Answer from the drawing. Dimensions are ordinates in mm from the lowest x, y and z of the part. A direction names the side the tool comes from. Coordinates: 2 decimals unless noted, no trailing zeros. Write each loop counter-clockwise with the first axis right and the second up, starting at its lowest first coordinate (ties: lowest second). Pieces come first, ordered by that corner, then holes.
(1) The part is cut by section B-B, the plane y = 42.5. Determine the outline of the cut face in (x, z) (1 decimal).
(2) Which of the six approach directions +Z, -Z, +X, -X, +Y, -Y give full straight-line access (tool end or side, diameter ignored) to the marked faces 5 and 6?
(3) The part is cut by section A-A, the plane z = 26.5. Determine the outline of the cut face in (x, y) (1 decimal).
(4) Straight lines are drawn through the part: line 1 along X through (y, z) = (20, 48) (1 decimal); line 2 along Y through (x, z) = (11, 48) (1 decimal); line 3 along Z through (x, y) = (25, 26). For each, find the intervals that lie inside material, in ascending order.
(5) Given pin 1 (5 mm diameter, centred on x = 21.5, y = 18, fed in from +Z), flat-ended and moving along its own axis, determine where the tip first touches the part or whether it passes through.
(6) The part is cut by section C-C, the plane x = 3. Determine the outline of the cut face in (y, z) (1 decimal), and give its area (3 significant figures).
(7) Determine the mould class of the marked faces 1, 2, 3 and 4 for opening direction Y: pulls with the +Y half, pulls with the -Y half, needs draft (parallel to the pull), parting line crosses it, or undercut.
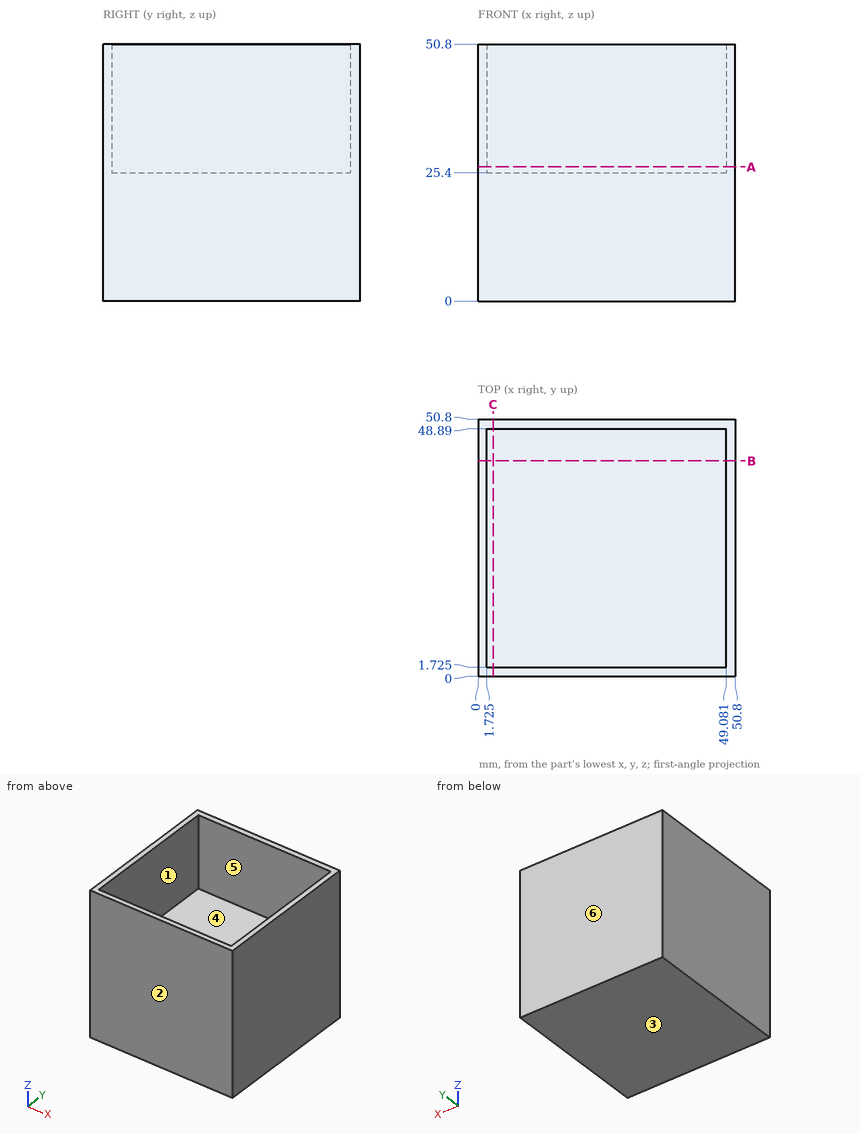
Computed:
1. outline: (0, 0) - (50.8, 0) - (50.8, 50.8) - (49.1, 50.8) - (49.1, 25.4) - (1.7, 25.4) - (1.7, 50.8) - (0, 50.8) - close
2. face 5: +Z
2. face 6: +Z, -Z, +X, -X, +Y
3. outline: (0, 0) - (50.8, 0) - (50.8, 50.8) - (0, 50.8) - close; hole (1.7, 1.7) - (49.1, 1.7) - (49.1, 48.9) - (1.7, 48.9) - close
4. line 1: x = 0 to 1.7, 49.1 to 50.8
4. line 2: y = 0 to 1.7, 48.9 to 50.8
4. line 3: z = 0 to 25.4
5. pin 1: stops at z = 25.4
6. outline: (0, 0) - (50.8, 0) - (50.8, 50.8) - (48.9, 50.8) - (48.9, 25.4) - (1.7, 25.4) - (1.7, 50.8) - (0, 50.8) - close
6. area: 1,380 mm2
7. face 1: undercut
7. face 2: pulls with the -Y half
7. face 3: needs draft
7. face 4: undercut
